Verification items for the finished model (mm, model axes). A direction names the side the tool comes from. Round coordinates to 2 decimals unless told otherwise and drop trailing zeros. Loops run counter-clockwise (first coordinate to the right, second up) from the corner with the lowest first, then second, coordinate; pieces in that order, holes last. Notation, with made-up numbers: (59, 9) - (99, 9) arc R22 ccw to (99, 17) - close; hole circle Ø3 at (59, -26). An arc over 180 degrees is marked (long way). Use CSV: the item, a comma, the result in double quotes.
```python
from build123d import *

# Parameters (mm, degrees)
SKETCH1_R               = 2.286
BOSS_EXTRUDE1_DEPTH     = 38.1
SKETCH2_W               = 10.922
SKETCH2_H               = 8.382
CUT_EXTRUDE1_DEPTH      = 6.08
CUT_EXTRUDE1_DEPTH_BACK = 6.08
SKETCH3_R               = 2.286
CUT_EXTRUDE2_DEPTH      = 6.08
CUT_EXTRUDE2_DEPTH_BACK = 6.08


with BuildPart() as part:
    # Sketch1 → Boss-Extrude1 (new body)
    with BuildSketch(Plane.XY):
        with BuildLine():
            Line((0, 5.08), (15.24, 5.08))
            ThreePointArc((15.24, 5.08), (23.912102448, 8.672102448), (20.32, 0))
            Line((20.32, 0), (0, 0))
            Line((0, 0), (0, 5.08))
        make_face()
        with Locations((20.32, 5.08)):
            Circle(SKETCH1_R, mode=Mode.SUBTRACT)
    extrude(amount=BOSS_EXTRUDE1_DEPTH)

    # Sketch2 → Cut-Extrude1 (cut, two sides)
    with BuildSketch(Plane(origin=(0, 5.08, 0), x_dir=(1, 0, 0), z_dir=(0, 1, 0))) as cut_extrude1_sk:
        with Locations((19.939, -11.303)):
            Rectangle(SKETCH2_W, SKETCH2_H)
        with Locations((19.939, -26.797)):
            Rectangle(SKETCH2_W, SKETCH2_H)
    extrude(amount=CUT_EXTRUDE1_DEPTH, mode=Mode.SUBTRACT)
    extrude(cut_extrude1_sk.sketch, amount=-CUT_EXTRUDE1_DEPTH_BACK, mode=Mode.SUBTRACT)

    # Sketch3 → Cut-Extrude2 (cut, two sides)
    with BuildSketch(Plane(origin=(0, 5.08, 0), x_dir=(1, 0, 0), z_dir=(0, 1, 0))) as cut_extrude2_sk:
        with Locations((6.4516, -10.414)):
            Circle(SKETCH3_R)
        with Locations((6.4516, -27.686)):
            Circle(SKETCH3_R)
    extrude(amount=CUT_EXTRUDE2_DEPTH, mode=Mode.SUBTRACT)
    extrude(cut_extrude2_sk.sketch, amount=-CUT_EXTRUDE2_DEPTH_BACK, mode=Mode.SUBTRACT)


solid = part.part
```
1) Gauge pin test, flat ends, axial feed: pin 1 Ø10 at (x, z) = (18.5, 25.5) entering from -Y; pin 2 Ø4 at (y, z) = (1.5, 11) entering from +X; pin 3 Ø2.5 at (x, z) = (6.45, 27.69) entering from -Y; pin 4 Ø3 at (x, z) = (3.5, 11) entering from +Y. Record the tip position at first contact, or that the pin passes through.
Returned:
pin 1,"stops at y = 0"
pin 2,"stops at x = 14.48"
pin 3,"passes through"
pin 4,"stops at y = 5.08"
2) Cross-section at A-A, the plane y = 3.75. Record the cut outline in (x, z).
Returned:
outline,"(0, 0) - (18.46, 0) - (18.46, 7.11) - (14.48, 7.11) - (14.48, 15.49) - (18.46, 15.49) - (18.46, 22.61) - (14.48, 22.61) - (14.48, 30.99) - (18.46, 30.99) - (18.46, 38.1) - (0, 38.1) - close; (22.18, 0) - (25.22, 0) - (25.22, 7.11) - (22.18, 7.11) - close; (22.18, 15.49) - (25.22, 15.49) - (25.22, 22.61) - (22.18, 22.61) - close; (22.18, 30.99) - (25.22, 30.99) - (25.22, 38.1) - (22.18, 38.1) - close; hole circle Ø4.57 at (6.45, 10.41); hole circle Ø4.57 at (6.45, 27.69)"
3) Cross-section at D-D, the plane y = 9. Record the cut outline in (x, z).
Returned:
outline,"(17.09, 0) - (23.55, 0) - (23.55, 7.11) - (17.09, 7.11) - close; (17.09, 15.49) - (23.55, 15.49) - (23.55, 22.61) - (17.09, 22.61) - close; (17.09, 30.99) - (23.55, 30.99) - (23.55, 38.1) - (17.09, 38.1) - close"
4) Access from +Z, -Z, +X, -X, +Y, -Y to the whole of each face (thin tool, end or side, straight path). Record for faces 1 (the face through (19, 3, 7.112)), 2 (the face through (10, 0, 19)).
Returned:
face 1,"+X, +Y, -Y"
face 2,"+Z, -Z, +X, -X, -Y"
5) Cross-section at C-C, the plane x = 18.75. Record the cut outline in (y, z).
Returned:
outline,"(0, 0) - (3.42, 0) - (3.42, 7.11) - (0, 7.11) - close; (0, 15.49) - (3.42, 15.49) - (3.42, 22.61) - (0, 22.61) - close; (0, 30.99) - (3.42, 30.99) - (3.42, 38.1) - (0, 38.1) - close; (6.74, 0) - (9.91, 0) - (9.91, 7.11) - (6.74, 7.11) - close; (6.74, 15.49) - (9.91, 15.49) - (9.91, 22.61) - (6.74, 22.61) - close; (6.74, 30.99) - (9.91, 30.99) - (9.91, 38.1) - (6.74, 38.1) - close"
6) Cross-section at B-B, the plane z = 29. Record the cut outline in (x, y).
Returned:
outline,"(0, 0) - (4.58, 0) - (4.58, 5.08) - (0, 5.08) - close; (8.32, 0) - (14.48, 0) - (14.48, 5.08) - (8.32, 5.08) - close"
7) Thickness scan on probe 1 along Z at (x, y) = (14.75, 2.5); probe 2 along Y at (x, z) = (20.32, 3.25); probe 3 along Y at (x, z) = (3, 18). Record the ranges inside material, lowest first. Write a range as [from, to].
Returned:
probe 1,"z = [0, 7.11], [15.49, 22.61], [30.99, 38.1]"
probe 2,"y = [0, 2.79], [7.37, 10.16]"
probe 3,"y = [0, 5.08]"
8) Mould release check, pull along Y, two halves, no side actions. Record for faces 3 (the face through (14.478, 3, 27)), 4 (the face through (22.43, 4.2, 34.49)), 5 (the face through (8, 5.08, 19)): +Y half, -Y half, draft (parallel to the pull), parting line (faces both ways), or undercut.
Returned:
face 3,"draft"
face 4,"undercut"
face 5,"+Y half"
